Can you work these out from the drawing? Everything is in mm from the part's minimum corner. A direction names the side the tool comes from. Give positions to 0.01 mm unless a question says otherwise; leave off trailing zeros. Order: outer loops, then holes, each group sorted by start corner. A loop starts at its lowest first (then second) coordinate and runs counter-clockwise, first axis right, second up. Notation, with made-up numbers: (57, 21) - (102, 21) arc R15 cw to (102, 43) - close; hole circle Ø7 at (-33, 12). An arc over 180 degrees is marked (long way). Answer as a JSON object with one key per item and string values.
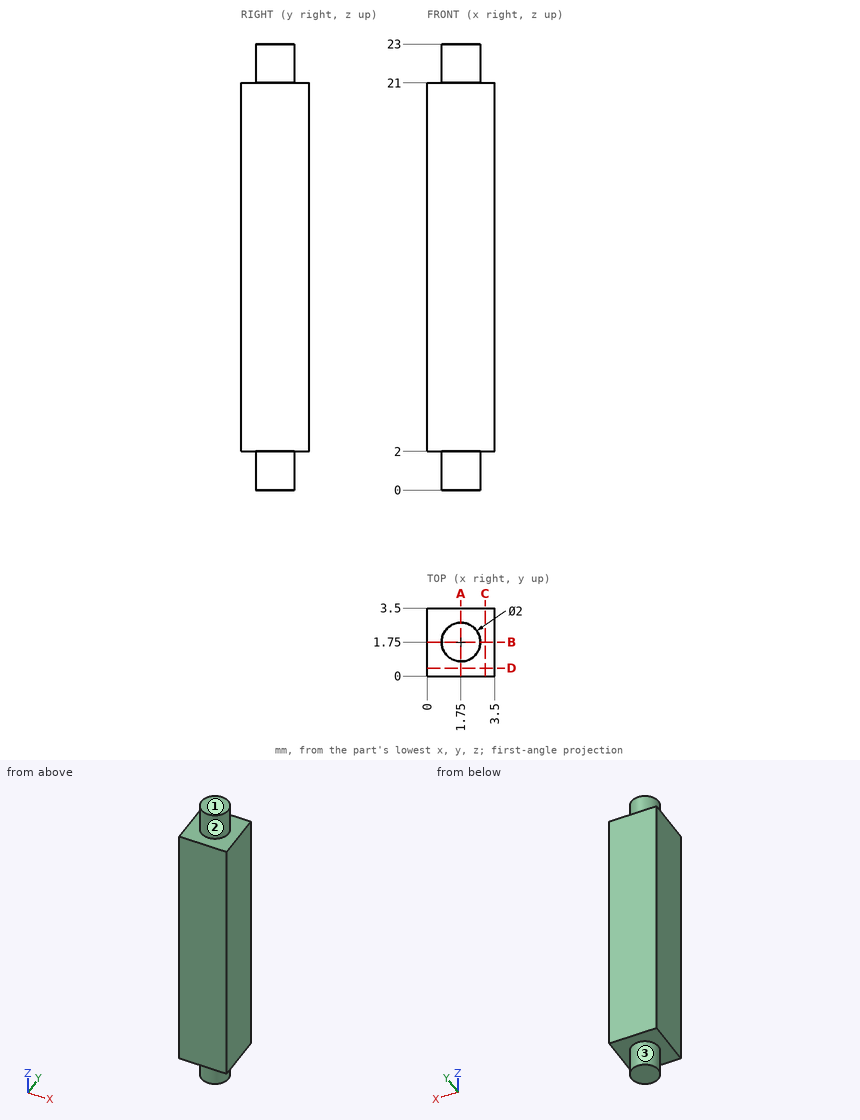
Q1. If we section it at C-C, the plane x = 3: Please give me the cut outline in (y, z), then the cut area to 3 significant figures.
Recorded:
{"outline": "(0, 2) - (3.5, 2) - (3.5, 21) - (0, 21) - close", "area": "66.5 mm^2"}
Q2. Which directions (+Z, -Z, +X, -X, +Y, -Y) give clear straight access to the entire face, cutting with the end or side of a thin tool? Please do the marked faces 1, 2 and 3.
Recorded:
{"face 1": "+Z, +X, -X, +Y, -Y", "face 2": "+Z", "face 3": "-Z"}
Q3. If we section it at A-A, the plane x = 1.75: Please give me the cut outline in (y, z).
Recorded:
{"outline": "(0, 2) - (0.75, 2) - (0.75, 0) - (2.75, 0) - (2.75, 2) - (3.5, 2) - (3.5, 21) - (2.75, 21) - (2.75, 23) - (0.75, 23) - (0.75, 21) - (0, 21) - close"}
Q4. I need wall thicknesses on L1, parallel to Z at x = 1, y = 0.2. Which ranges of the line are inside material? Lowest first, please.
Recorded:
{"L1": "z = 2 to 21"}
